```python
from build123d import *

# Parameters (mm, degrees)
F0_W     = 101.6
F0_H     = 101.6
F1_DEPTH = 25.4
F2_R     = 5.08
F3_R     = 5.08
F4_R     = 5.08
F5_R     = 5.08
F7_D     = 10.31875


# Not quite as in the source:
# - a length typed as a fraction of an inch, garbled in the dataset ("3 / 203.2 mm" for 3/8 in), is restored


with BuildPart() as f1:
    # F0 (on Top) → F1 (new body)
    with BuildSketch(Plane.XY):
        with Locations((-24.6530866301, 19.163233228)):
            Rectangle(F0_W, F0_H)
    extrude(amount=F1_DEPTH)

    # F2
    f2_edges = [f1.edges().sort_by_distance(p)[0] for p in [
        (-75.453087, 69.963233, 12.7),
    ]]
    fillet(f2_edges, radius=F2_R)

    # F3
    f3_edges = [f1.edges().sort_by_distance(p)[0] for p in [
        (-75.453087, -31.636767, 12.7),
    ]]
    fillet(f3_edges, radius=F3_R)

    # F4
    f4_edges = [f1.edges().sort_by_distance(p)[0] for p in [
        (26.146913, 69.963233, 12.7),
    ]]
    fillet(f4_edges, radius=F4_R)

    # F5
    f5_edges = [f1.edges().sort_by_distance(p)[0] for p in [
        (26.146913, -31.636767, 12.7),
    ]]
    fillet(f5_edges, radius=F5_R)

    # F7 (through all)
    with Locations(Plane.XY.offset(25.4)):
        with Locations((-24.9434951693, 15.3265725821)):
            Hole(F7_D / 2)


solid = f1.part
```
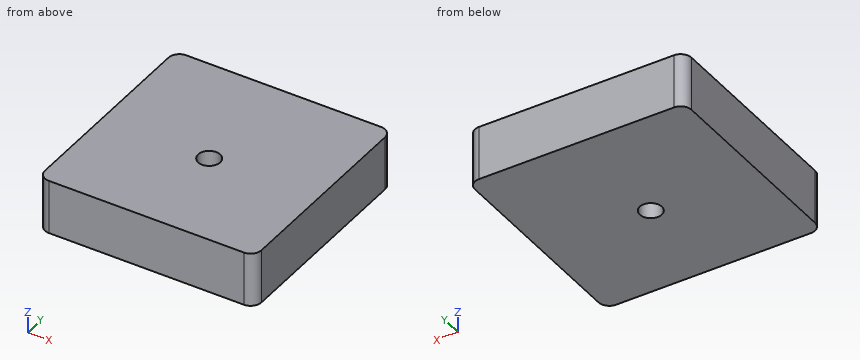
Source: CAD feature listing. Evaluate the final solid. Frame: model axes, mm. Coordinates: 2 decimals unless noted, no trailing zeros. Write each loop counter-clockwise with the first axis right and the second up, starting at its lowest first coordinate (ties: lowest second). Pieces come first, ordered by that corner, then holes. Notation, with made-up numbers: (74, 21) -> (110, 21) arc R28 ccw to (110, 52) -> close; hole circle Ø8 at (76, -26). An arc over 180 degrees is marked (long way). Return JSON: item names as keys, results as strings. Group by question number.
1) Ray query, line 1 along X through (y, z) = (65, 11.75); line 2 along Y through (x, z) = (-26.5, 4.25). Return the intervals inside material, ascending.
2) Section query B-B, the plane x = -26.5. Return loops of the section in (y, z), plus the area to 3 significant figures.
3) Section query A-A, the plane y = 11.5. Return loops of the section in (x, z), plus the area to 3 significant figures.
From the geometry:
{
 "1": {"line 1": "-75.45 to 26.15", "line 2": "-31.64 to 10.41, 20.25 to 69.96"},
 "2": {"outline": "(-31.64, 0) -> (10.41, 0) -> (10.41, 25.4) -> (-31.64, 25.4) -> close; (20.25, 0) -> (69.96, 0) -> (69.96, 25.4) -> (20.25, 25.4) -> close", "area": "2,330 mm²"},
 "3": {"outline": "(-75.45, 0) -> (-28.4, 0) -> (-28.4, 25.4) -> (-75.45, 25.4) -> close; (-21.48, 0) -> (26.15, 0) -> (26.15, 25.4) -> (-21.48, 25.4) -> close", "area": "2,400 mm²"}
}
